from build123d import *

# Parameters (mm, degrees)
IZIM1_W                              = 100
IZIM1_H                              = 50
IZIM1_R                              = 2.476303865
IZIM1_R_2                            = 9.5
IZIM1_R_3                            = 2.283039358
Y_KSEKLIK_EKSTR_ZYON1_DEPTH          = 8
M5_HELISARMAL_I_IN_Z_VANA_MATKAB_1_D = 5.2
M5_HELISARMAL_I_IN_Z_VANA_MATKAB_2_D = 5.2
KES_EKSTR_ZYON1_DEPTH                = 10


with BuildPart() as part:
    # Çizim1 → Yükseklik-Ekstrüzyon1 (new body)
    # profile 1 of 6: a face of its own
    with BuildSketch(Plane.XY):
        with Locations((91.850220264, -26.688693098)):
            Rectangle(IZIM1_W, IZIM1_H)
        with Locations((131.850220264, -41.688693098)):
            Circle(IZIM1_R, mode=Mode.SUBTRACT)
        with Locations((111.850220264, -26.688693098)):
            Circle(IZIM1_R_2, mode=Mode.SUBTRACT)
        with Locations((131.850220264, -11.688693098)):
            Circle(IZIM1_R_3, mode=Mode.SUBTRACT)
    # profile 2 of 6: a face of its own
    with BuildSketch(Plane.XY):
        with Locations((-8.149779736, -26.688693098)):
            Rectangle(IZIM1_W, IZIM1_H)
        with Locations((-48.149779736, -41.688693098)):
            Circle(IZIM1_R, mode=Mode.SUBTRACT)
        with Locations((-28.149779736, -26.688693098)):
            Circle(IZIM1_R_2, mode=Mode.SUBTRACT)
        with Locations((-48.149779736, -11.688693098)):
            Circle(IZIM1_R_3, mode=Mode.SUBTRACT)
    # profile 3 of 6: a face of its own
    with BuildSketch(Plane.XY):
        with Locations((-48.149779736, -11.688693098)):
            Circle(IZIM1_R_3)
    # profile 4 of 6: a face of its own
    with BuildSketch(Plane.XY):
        with Locations((-48.149779736, -41.688693098)):
            Circle(IZIM1_R)
    # profile 5 of 6: a face of its own
    with BuildSketch(Plane.XY):
        with Locations((131.850220264, -11.688693098)):
            Circle(IZIM1_R_3)
    # profile 6 of 6: a face of its own
    with BuildSketch(Plane.XY):
        with Locations((131.850220264, -41.688693098)):
            Circle(IZIM1_R)
    extrude(amount=Y_KSEKLIK_EKSTR_ZYON1_DEPTH)

    # M5 Helisarmal için Zıvana matkabı1 (through all)
    with Locations(Plane.XY.offset(8)):
        with Locations((-48.149779736, -11.688693098), (-48.149779736, -41.688693098), (131.850220264, -41.688693098), (131.850220264, -11.688693098)):
            Hole(M5_HELISARMAL_I_IN_Z_VANA_MATKAB_1_D / 2)

    # M5 Helisarmal için Zıvana matkabı2 (through all)
    with Locations(Plane(origin=(-18.149779736, -41.688693098, 8), x_dir=(1, 0, 0), z_dir=(0, 0, 1))):
        with Locations((0, 0), (120, 0)):
            Hole(M5_HELISARMAL_I_IN_Z_VANA_MATKAB_2_D / 2)

    # Çizim7 → Kes-Ekstrüzyon1 (cut)
    with BuildSketch(Plane.XY.offset(8)):
        with BuildLine():
            ThreePointArc((51.350220264, -26.688693098), (48.567734686, -19.971178677), (41.850220264, -17.188693098))
            Line((41.850220264, -17.188693098), (41.850220264, -36.188693098))
            ThreePointArc((41.850220264, -36.188693098), (48.567734686, -33.40620752), (51.350220264, -26.688693098))
        make_face()
        with BuildLine():
            Line((41.850220264, -36.188693098), (41.850220264, -17.188693098))
            ThreePointArc((41.850220264, -17.188693098), (32.350220264, -26.688693098), (41.850220264, -36.188693098))
        make_face()
    extrude(amount=-KES_EKSTR_ZYON1_DEPTH, mode=Mode.SUBTRACT)


solid = part.part
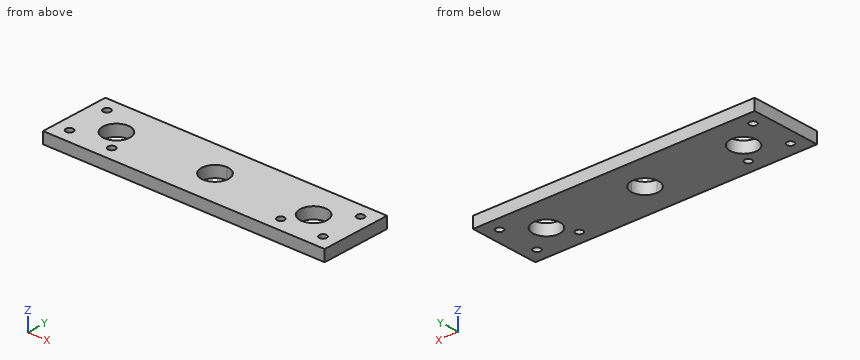
Source: CAD feature listing. Evaluate the final solid. Frame: model axes, mm. Give positions to 0.01 mm unless a question says otherwise; leave off trailing zeros. Write each loop counter-clockwise with the first axis right and the second up, starting at its lowest first coordinate (ties: lowest second). Pieces come first, ordered by that corner, then holes. Notation, with made-up numbers: M 23.5,-20 L 58.5,-20 A21 ccw 58.5,11 Z; hole C 35,26.5 d7. An arc over 180 degrees is marked long. Return JSON: item names as keys, results as strings. Group by question number.
1) Cut plane B-B, the plane z = 2. Give the number of separate pieces and of enclosed holes in the cut face, then the cut area to 3 significant figures.
2) Ray query, L1, parallel to X at y = -26, z = 5.75; L2, parallel to X at y = -14, z = 5; L3, parallel to X at y = -25, z = 7. Return the intervals inside material, ascending.
3) Cut plane A-A, the plane y = -22.5. Output: boundary loops of the cut face in (x, z), then the cut area to 3 significant figures.
4) Cut plane D-D, the plane y = -34. Output: boundary loops of the cut face in (x, z).
5) First-contact query: pin 1 Ø3 at (x, y) = (-18.15, -41.69) entering from +Z. Flat tip, straight axial feed; report the tip coordinate or a pass-through.
6) Cut plane C-C, the plane x = -28. Output: boundary loops of the cut face in (y, z).
Data:
{
 "1": {"separate pieces": "1", "enclosed holes": "9", "area": "9,020 mm²"},
 "2": {"L1": "x = -58.15 to -37.62, -18.67 to 32.38, 51.33 to 102.38, 121.33 to 141.85", "L2": "x = -58.15 to -49.34, -46.96 to 130.66, 133.04 to 141.85", "L3": "x = -58.15 to -37.5, -18.8 to 32.5, 51.2 to 102.5, 121.2 to 141.85"},
 "3": {"outline": "M -58.15,0 L -36.68,0 L -36.68,8 L -58.15,8 Z; M -19.62,0 L 33.32,0 L 33.32,8 L -19.62,8 Z; M 50.38,0 L 103.32,0 L 103.32,8 L 50.38,8 Z; M 120.38,0 L 141.85,0 L 141.85,8 L 120.38,8 Z", "area": "1,190 mm²"},
 "4": {"outline": "M -58.15,0 L -34.22,0 L -34.22,8 L -58.15,8 Z; M -22.08,0 L 35.78,0 L 35.78,8 L -22.08,8 Z; M 47.92,0 L 105.78,0 L 105.78,8 L 47.92,8 Z; M 117.92,0 L 141.85,0 L 141.85,8 L 117.92,8 Z"},
 "5": {"pin 1": "passes through"},
 "6": {"outline": "M -51.69,0 L -36.19,0 L -36.19,8 L -51.69,8 Z; M -17.19,0 L -1.69,0 L -1.69,8 L -17.19,8 Z"}
}
